Geometry check sheet. Reference: the model listing, model coordinates, mm. Face numbers are marked on the shaded views. A direction names the side the tool comes from. Coordinates: 2 decimals unless noted, no trailing zeros. Loops run counter-clockwise (first coordinate to the right, second up) from the corner with the lowest first, then second, coordinate; pieces in that order, holes last. Notation, with made-up numbers: (78.5, 15.5) - (124.5, 15.5) arc R18 cw to (124.5, 27.5) - close; hole circle Ø2 at (82.5, 56). An arc over 180 degrees is marked (long way). Write item = value, one per line. Start each with the question number.
from build123d import *

# Parameters (mm, degrees)
F0_R     = 10.16
F1_DEPTH = 15.7734
F2_DEPTH = 24.4602
F3_R     = 3.302


with BuildPart() as f1:
    # F0 (on Top) → F1 (new body)
    with BuildSketch(Plane.XY):
        with BuildLine():
            ThreePointArc((-23.198551, -28.126541), (-6.325173, -18.336262), (0.333802, 0))
            ThreePointArc((0.333802, 0), (-6.325173, 18.336262), (-23.198551, 28.126541))
            ThreePointArc((-23.198551, 28.126541), (-56.816198, 0), (-23.198551, -28.126541))
        make_face()
        with BuildLine():
            ThreePointArc((-14.781716, -4.793226), (-42.528698, 0), (-14.781716, 4.793226))
            Line((-14.781716, 4.793226), (-6.636774, 4.793226))
            Line((-6.636774, 4.793226), (-6.636774, -4.793226))
            Line((-6.636774, -4.793226), (-14.781716, -4.793226))
        make_face(mode=Mode.SUBTRACT)
        with BuildLine():
            ThreePointArc((-23.198551, 28.126541), (-6.325173, 18.336262), (0.333802, 0))
            ThreePointArc((0.333802, 0), (-6.325173, -18.336262), (-23.198551, -28.126541))
            Line((-23.198551, -28.126541), (29.095567, -18.751028))
            ThreePointArc((29.095567, -18.751028), (6.683802, 0), (29.095567, 18.751028))
            Line((29.095567, 18.751028), (-23.198551, 28.126541))
        make_face()
        with BuildLine():
            ThreePointArc((44.783802, 0), (40.344485, 12.224174), (29.095567, 18.751028))
            ThreePointArc((29.095567, 18.751028), (6.683802, 0), (29.095567, -18.751028))
            ThreePointArc((29.095567, -18.751028), (40.344485, -12.224174), (44.783802, 0))
        make_face()
        with Locations((25.733802, 0)):
            Circle(F0_R, mode=Mode.SUBTRACT)
        with BuildLine():
            Line((-6.636774, 4.793226), (-14.781716, 4.793226))
            ThreePointArc((-14.781716, 4.793226), (-42.528698, 0), (-14.781716, -4.793226))
            Line((-14.781716, -4.793226), (-6.636774, -4.793226))
            Line((-6.636774, -4.793226), (-6.636774, 4.793226))
        make_face()
    extrude(amount=-F1_DEPTH)

    # F0 (on Top) → F2 (join)
    with BuildSketch(Plane.XY):
        with BuildLine():
            ThreePointArc((-23.198551, -28.126541), (-6.325173, -18.336262), (0.333802, 0))
            ThreePointArc((0.333802, 0), (-6.325173, 18.336262), (-23.198551, 28.126541))
            ThreePointArc((-23.198551, 28.126541), (-56.816198, 0), (-23.198551, -28.126541))
        make_face()
        with BuildLine():
            ThreePointArc((-14.781716, -4.793226), (-42.528698, 0), (-14.781716, 4.793226))
            Line((-14.781716, 4.793226), (-6.636774, 4.793226))
            Line((-6.636774, 4.793226), (-6.636774, -4.793226))
            Line((-6.636774, -4.793226), (-14.781716, -4.793226))
        make_face(mode=Mode.SUBTRACT)
    extrude(amount=F2_DEPTH)

    # F3
    f3_edges = [f1.edges().sort_by_distance(p)[0] for p in [
        (-33.283845, 28.126541, 24.4602),
    ]]
    fillet(f3_edges, radius=F3_R)


solid = f1.part
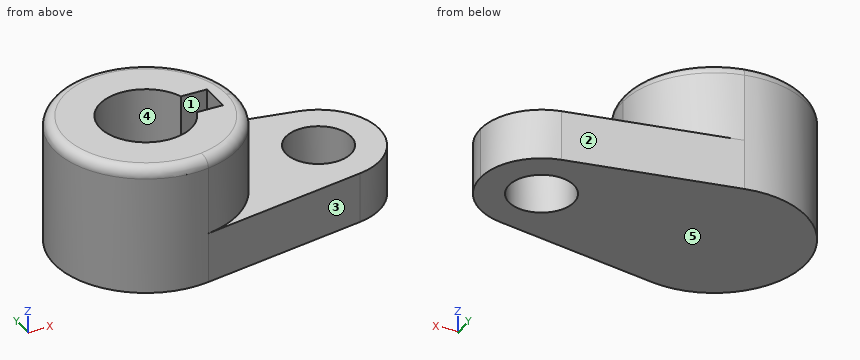
(1) Tool access check on the marked faces 1 and 2. Record the directions out of +Z, -Z, +X, -X, +Y, -Y that give a thin tool (end or side, any length) a straight path to the whole face; none if there is none.
(2) Sectioned sample at C-C on z = -6. Enter the section's corners in (x, y) (3 decimals).
(3) Scan lines: line 1 (Y direction, x = -29, z = 13); line 2 (X direction, y = 0, z = 13); line 3 (Z direction, x = -35, y = -8.5). Record each from-to range of solid material in increasing order.
(4) Sectioned sample at B-B on x = 26. Enter the section's corners in (y, z).
(5) Depth check by flat-ended pin: pin 1 (2 mm diameter, centred on x = -17, z = 15, fed in from -Y); pin 2 (3 mm diameter, centred on y = -0.5, z = 9, fed in from -X); pin 3 (6.5 mm diameter, centred on x = -11, z = 10, fed in from +Y). Enter the tip coordinate at first touch or a pass-through.
(6) Draft check along Y on the marked faces 3, 4 and 5. Enter one of: pulls with the +Y half, pulls with the -Y half, needs draft (parallel to the pull), parting line crosses it, or undercut.
Working result:
q1.face_1 = +Z
q1.face_2 = +Z, -Z, +X, +Y
q2.outline = (-23.199, -28.127) - (29.096, -18.751) arc R19.05 ccw to (44.784, 0) arc R19.05 ccw to (29.096, 18.751) - (-23.199, 28.127) arc R28.575 ccw (long way) to start; hole circle Ø20.32 at (25.734, 0)
q3.line_1 = -28.56 to -14.27, 14.27 to 28.56
q3.line_2 = -56.82 to -42.53, -6.64 to 0.33
q3.line_3 = -15.77 to 0
q4.outline = (-19.31, -15.77) - (-10.16, -15.77) - (-10.16, 0) - (-19.31, 0) - close; (10.16, -15.77) - (19.31, -15.77) - (19.31, 0) - (10.16, 0) - close
q5.pin_1 = -26.68
q5.pin_2 = -56.82
q5.pin_3 = 24.92
q6.face_3 = pulls with the -Y half
q6.face_4 = undercut
q6.face_5 = needs draft
